Study the drawing (mm; zero at the part's minimum x, y, z) and answer. A direction names the side the tool comes from. Coordinates: 2 decimals unless noted, no trailing zeros. Order: outer loops, then holes, each group sorted by start corner. A loop starts at its lowest first (then second) coordinate and runs counter-clockwise, first axis right, second up.
1. The part is cut by section A-A, the plane z = 3.25. Give the vertices of the cut face in (x, y).
2. The part is cut by section B-B, the plane x = 4. Give the vertices of the cut face in (y, z), then the cut area to 3 significant figures.
3. A tool of negligible diameter and unlimited length cuts with its end or side. For the marked faces 4 and 5, from which of +Z, -Z, +X, -X, +Y, -Y can it reach the whole face along a straight path? Write none if from no direction.
4. Determine the mould class of the marked faces 1, 2 and 3 for opening direction X: +X half, -X half, draft (parallel to the pull), parting line (faces both ways), or undercut.
5. Flat-ended cylindrical pins translate along their axes: pin 1 Ø0.8 at (x, y) = (3.5, 3.5) entering from -Z; pin 2 Ø3.5 at (x, y) = (5.5, 4) entering from -Z; pin 3 Ø1 at (y, z) = (2, 2) entering from -X; pin 4 Ø1 at (x, z) = (2, 5.5) entering from -Y. Find the tip coordinate at first contact, or state that the pin passes through.
6. Find the intervals of material crossed by probe 1 along Y at (x, z) = (4, 3.5); probe 2 along Y at (x, z) = (3.5, 1.5); probe 3 along X at (y, z) = (5, 1.75), in increasing order.
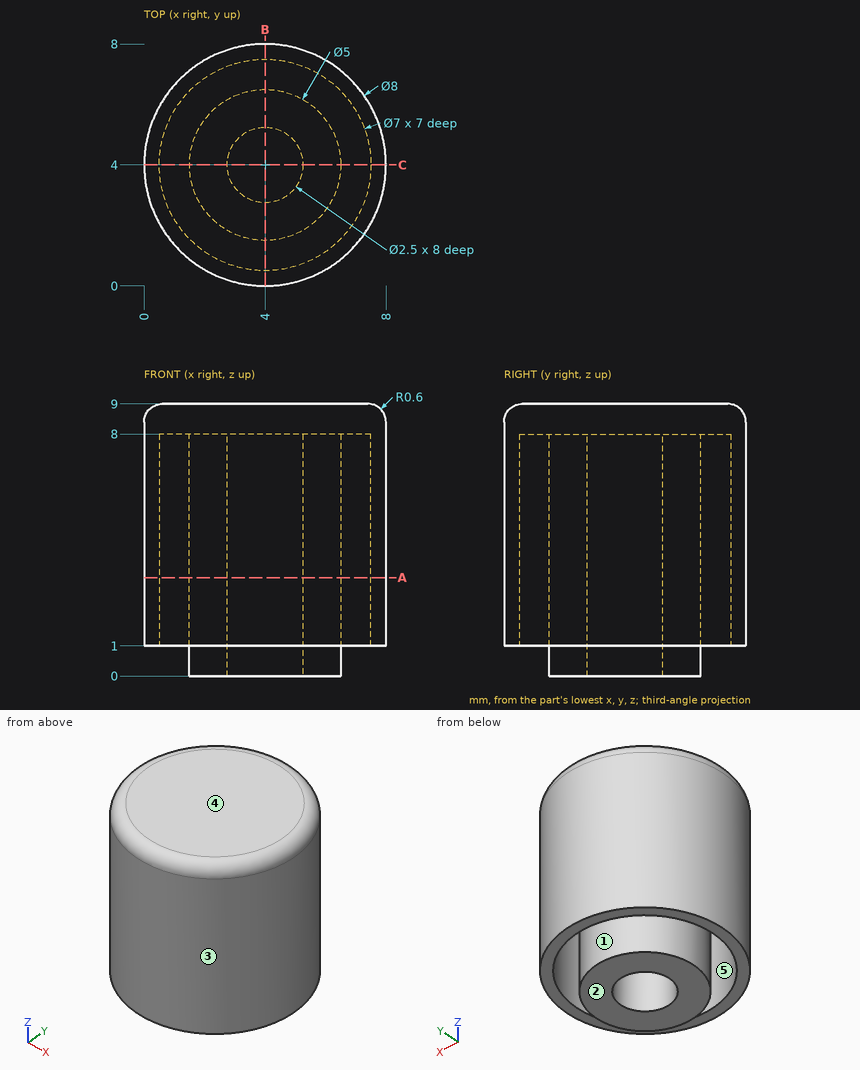
Geometry says:
1. outline: circle Ø8 at (4, 4); circle Ø5 at (4, 4); hole circle Ø7 at (4, 4); hole circle Ø2.5 at (4, 4)
2. outline: (0, 1) - (0.5, 1) - (0.5, 8) - (1.5, 8) - (1.5, 0) - (2.75, 0) - (2.75, 8) - (5.25, 8) - (5.25, 0) - (6.5, 0) - (6.5, 8) - (7.5, 8) - (7.5, 1) - (8, 1) - (8, 8.4) arc R0.6 ccw to (7.4, 9) - (0.6, 9) arc R0.6 ccw to (0, 8.4) - close
2. area: 34.8 mm2
3. face 4: +Z, +X, -X, +Y, -Y
3. face 5: -Z
4. face 1: undercut
4. face 2: draft
4. face 3: parting line
5. pin 1: stops at z = 8
5. pin 2: stops at z = 0
5. pin 3: stops at x = 0.29
5. pin 4: stops at y = 0.29
6. probe 1: y = 0 to 0.5, 1.5 to 2.75, 5.25 to 6.5, 7.5 to 8
6. probe 2: y = 0.03 to 0.54, 1.55 to 2.85, 5.15 to 6.45, 7.46 to 7.97
6. probe 3: x = 0.13 to 0.65, 1.71 to 3.25, 4.75 to 6.29, 7.35 to 7.87
